```python
from build123d import *

# Parameters (mm, degrees)
F1_DEPTH = 2
F2_DEPTH = 5
F3_DEPTH = 2
F4_R     = 1
F5_D     = 2


with BuildPart() as f1:
    # F0 (on Top) → F1 (new body)
    with BuildSketch(Plane.XY):
        with BuildLine():
            ThreePointArc((4.582575695, 2), (4.8945315647, 1.0215482184), (5, 0))
            Line((5, 0), (10, 0))
            Line((10, 0), (10, 2))
            Line((10, 2), (4.582575695, 2))
        make_face()
    extrude(amount=F1_DEPTH)

    # F0 (on Top) → F2 (join)
    with BuildSketch(Plane.XY):
        with BuildLine():
            ThreePointArc((4.582575695, 2), (-4.8945315647, -1.0215482184), (5, 0))
            ThreePointArc((5, 0), (4.8945315647, 1.0215482184), (4.582575695, 2))
        make_face()
    extrude(amount=F2_DEPTH)

    # F0 (on Top) → F3 (join, symmetric)
    with BuildSketch(Plane.XY):
        Polygon((10, 2), (10, 0), (15.196, 0), (15.196, 1), (10, 4), align=None)
    extrude(amount=F3_DEPTH, both=True)

    # F4
    f4_edges = [f1.edges().sort_by_distance(p)[0] for p in [
        (10, 4, 0),
    ]]
    fillet(f4_edges, radius=F4_R)

    # F5 (through all)
    with Locations(Plane(origin=(0, 0, 0), x_dir=(1, 0, 0), z_dir=(0, 0, -1))):
        with Locations((0, 0)):
            Hole(F5_D / 2)


solid = f1.part
```
Design review of the part built by this model. Coordinates are the model's own, in mm. A direction names the side the tool comes from. Give positions to 0.01 mm unless a question says otherwise; leave off trailing zeros. Write each loop counter-clockwise with the first axis right and the second up, starting at its lowest first coordinate (ties: lowest second). Pieces come first, ordered by that corner, then holes.
(1) Tool access review of faces 1 (the face through (10, 1, -1)), 2 (the face through (7, 2, 1)), 3 (the face through (11, 0, 0)), 4 (the face through (15.196, 0.5, 0)), 5 (the face through (-0.1, 1.2, 5)): name each direction out of +Z, -Z, +X, -X, +Y, -Y from which nothing blocks a thin tool from reaching the whole face with its end or side.
Checked values:
face 1: -Z, +Y
face 2: +Z, -Z, +Y
face 3: +Z, -Z, +X, -Y
face 4: +Z, -Z, +X, +Y, -Y
face 5: +Z, +X, -X, +Y, -Y
(2) Add section D-D (z = -1.25). Give the boundary of the cut face in (x, y), and give its area (3 significant figures).
Checked values:
outline: (10, 0) - (15.2, 0) - (15.2, 1) - (11.5, 3.13) arc R1 ccw to (10, 2.27) - close
area: 12.3 mm2
(3) Wall thickness on line 1 along Y through (x, z) = (0, 3.45); line 2 along Z through (x, y) = (12.25, 1.5); line 3 along Y through (x, z) = (9, 1.75): over which ranges is each line inside the solid? List them lowest first.
Checked values:
line 1: y = -5 to -1, 1 to 5
line 2: z = -2 to 2
line 3: y = 0 to 2
(4) Add section A-A (z = 0.75). Give the boundary of the cut face in (x, y).
Checked values:
outline: (4.58, 2) arc R5 ccw (long way) to (5, 0) - (15.2, 0) - (15.2, 1) - (11.5, 3.13) arc R1 ccw to (10, 2.27) - (10, 2) - close; hole circle Ø2 at (0, 0)
(5) Add section B-B (x = 0). Give the boundary of the cut face in (y, z), and give its area (3 significant figures).
Checked values:
outline: (-5, 0) - (-1, 0) - (-1, 5) - (-5, 5) - close; (1, 0) - (5, 0) - (5, 5) - (1, 5) - close
area: 40.0 mm2
(6) Clearance check with flat-ended pins moving along their axes: pin 1 Ø2 at (x, z) = (6.5, 1) entering from +Y; pin 2 Ø3 at (x, z) = (11.5, 2.5) entering from +Y; pin 3 Ø1 at (x, y) = (9.5, 2) entering from +Z; pin 4 Ø3 at (x, y) = (5, 1) entering from +Z. State where each tip first meets the part, or that it passes through.
Checked values:
pin 1: stops at y = 2
pin 2: stops at y = 3.27
pin 3: stops at z = 2
pin 4: stops at z = 5
(7) Mouldability with a two-part tool opening along X and no side actions: class faces 6 (the face through (13.374, 2.052, 0.028)), 7 (the face through (0, 1, 3)), 8 (the face through (1, -1, 0)) as +X half, -X half, draft (parallel to the pull), parting line (faces both ways), or undercut.
Checked values:
face 6: +X half
face 7: undercut
face 8: draft
(8) Add section C-C (y = 0.25). Give the boundary of the cut face in (x, z), and give its area (3 significant figures).
Checked values:
outline: (-4.99, 0) - (-0.97, 0) - (-0.97, 5) - (-4.99, 5) - close; (0.97, 0) - (10, 0) - (10, -2) - (15.2, -2) - (15.2, 2) - (4.99, 2) - (4.99, 5) - (0.97, 5) - close
area: 71.1 mm2
